from build123d import *

# Parameters (mm, degrees)
SKETCH1_R           = 0.5
BOSS_EXTRUDE1_DEPTH = 12
CUT_EXTRUDE1_DEPTH  = 1
CHAMFER1_SIZE       = 0.05
SCALE1_SCALE        = 1.9329
SCALE2_SCALE        = 1.5


with BuildPart() as part:
    # Sketch1 → Boss-Extrude1 (new body)
    with BuildSketch(Plane.XY):
        Circle(SKETCH1_R)
    extrude(amount=BOSS_EXTRUDE1_DEPTH)

    # Sketch2 → Cut-Extrude1 (cut)
    with BuildSketch(Plane.XY.offset(12)):
        Polygon((0.369541813, -0.215248582), (0.371181646, 0.212408307), (0.001639833, 0.427656888), (-0.369541813, 0.215248582), (-0.371181646, -0.212408307), (-0.001639833, -0.427656888), align=None)
    extrude(amount=-CUT_EXTRUDE1_DEPTH, mode=Mode.SUBTRACT)

    # Chamfer1
    chamfer1_edges = [part.edges().sort_by_distance(p)[0] for p in [
        (0.18395099, -0.321452735, 12),
        (0.370361729, -0.001420137, 12),
        (0.18641074, 0.320032598, 12),
        (-0.18395099, 0.321452735, 12),
        (-0.370361729, 0.001420137, 12),
        (-0.18641074, -0.320032598, 12),
    ]]
    chamfer(chamfer1_edges, length=CHAMFER1_SIZE)


with BuildPart() as part_1:
    # Scale1: scaled about (0, 0, 5.705631977)
    add(part.part.scale(SCALE1_SCALE).moved(Location((0, 0, -5.322784071))))


with BuildPart() as part_2:
    # Scale2: scaled about (0, 0, 5.705631977)
    add(part_1.part.scale(SCALE2_SCALE).moved(Location((0, 0, -2.852815989))))


solid = part_2.part
Work out the finished part from the listing and answer in its coordinate system (mm). Round coordinates to 2 decimals unless told otherwise and drop trailing zeros. Write each loop counter-clockwise with the first axis right and the second up, starting at its lowest first coordinate (ties: lowest second). Pieces come first, ordered by that corner, then holes. Notation, with made-up numbers: (42, -13) - (49, -13) arc R23 cw to (49, 22) - close; hole circle Ø8 at (74, -3.75). An arc over 180 degrees is marked (long way). Answer in a Markdown table with one row per item. Add a question column.
1. Find the intervals of material crossed by line 1 along X through (y, z) = (-0.1, 22); line 2 along Y through (x, z) = (-0.8, 4); line 3 along Z through (x, y) = (0.85, 0.05), in increasing order. Write a range as from..to.
2. Given pin 1 (1.1 mm diameter, centred on x = 0, y = 0.5, fed in from +Z), flat-ended and moving along its own axis, determine where the tip first touches the part or whether it passes through.
3. A cutting plane is placed at B-B, the plane y = 0. Determine the outline of the cut face in (x, z).
4. The mould has two halves that part along Y. Classify faces 1 (the flat face through (0, 0, -10.837)), 2 (the cylindrical face through (-1.15, -0.88, 6.32)), 3 (the flat face through (0.548, 0.924, 22.452)): +Y half, -Y half, draft (parallel to the pull), parting line (faces both ways), or undercut.
5. A cutting plane is placed at C-C, the plane x = 0.45. Determine the outline of the cut face in (y, z), and give its area (3 significant figures).
6. A cutting plane is placed at A-A, the plane z = 12. Determine the outline of the cut face in (x, y), and give its area (3 significant figures).
Worked out:
| question | item | result |
|---|---|---|
| 1 | line 1 | -1.45..-1.07, 1.07..1.45 |
| 1 | line 2 | -1.21..1.21 |
| 1 | line 3 | -10.84..21.06 |
| 2 | pin 1 | z = 21.06 |
| 3 | outline | (-1.45, -10.84) - (1.45, -10.84) - (1.45, 23.96) - (1.22, 23.96) - (1.07, 23.81) - (1.07, 21.06) - (-1.07, 21.06) - (-1.07, 23.81) - (-1.22, 23.96) - (-1.45, 23.96) - close |
| 4 | face 1 | draft |
| 4 | face 2 | parting line |
| 4 | face 3 | undercut |
| 5 | outline | (-1.38, -10.84) - (1.38, -10.84) - (1.38, 23.96) - (1.15, 23.96) - (0.98, 23.81) - (0.98, 21.06) - (-0.98, 21.06) - (-0.98, 23.81) - (-1.15, 23.96) - (-1.38, 23.96) - close |
| 5 | area | 90.2 mm^2 |
| 6 | outline | circle Ø2.9 at (0, 0) |
| 6 | area | 6.60 mm^2 |
